from build123d import *

# Parameters (mm, degrees)
SKETCH3_W                       = 3
SKETCH3_H                       = 10
BOSS_EXTRUDE1_DEPTH             = 15
SKETCH3_W_2                     = 9.160158842
BOSS_EXTRUDE1_2_DEPTH           = 15
BOSS_EXTRUDE1_3_DEPTH           = 15
SKETCH4_W                       = 22.820603272
SKETCH4_H                       = 10
BOSS_EXTRUDE2_DEPTH             = 3
SKETCH5_W                       = 22.820603272
SKETCH5_H                       = 10
BOSS_EXTRUDE3_DEPTH             = 3
SKETCH7_W                       = 16
SKETCH7_H                       = 14.76
BOSS_EXTRUDE4_DEPTH             = 10
SKETCH8_W                       = 6.35
SKETCH8_H                       = 35.2
CUT_EXTRUDE1_DEPTH              = 10
TAP_DRILL_FOR_M3X0_5_TAP1_D     = 2.5
TAP_DRILL_FOR_M3X0_5_TAP1_DEPTH = 10
TAP_DRILL_FOR_M3X0_5_TAP1_TIP   = 0.751075774
BOSS_EXTRUDE5_DEPTH             = 10
CUT_EXTRUDE4_DEPTH              = 319.166667347
CUT_EXTRUDE5_DEPTH              = 5
M4_START                        = -10.356969024
M4_CLEARANCE_SLOT1_DEPTH        = 5
FILLET4_R                       = 2


# Read off the part's stored shape, not the designer's step: M4 Clearance Slot1
with BuildPart() as part:
    # Sketch3 → Boss-Extrude1 (new body)
    with BuildSketch(Plane(origin=(-193.9, 0, 193.9), x_dir=(0.7071067811865475, 0, 0.7071067811865477), z_dir=(-0.7071067811865477, 0, 0.7071067811865475))):
        with Locations((-9.910301636, -10.356969024)):
            Rectangle(SKETCH3_W, SKETCH3_H)
    extrude(amount=-BOSS_EXTRUDE1_DEPTH)



with BuildPart() as body_2:
    # Sketch3 → Boss-Extrude1 2 (new body)
    with BuildSketch(Plane(origin=(-193.9, 0, 193.9), x_dir=(0.7071067811865475, 0, 0.7071067811865477), z_dir=(-0.7071067811865477, 0, 0.7071067811865475))):
        with Locations((0, -10.356969024)):
            Rectangle(SKETCH3_W_2, SKETCH3_H)
    extrude(amount=-BOSS_EXTRUDE1_2_DEPTH)


with BuildPart() as body_3:
    # Sketch3 → Boss-Extrude1 3 (new body)
    with BuildSketch(Plane(origin=(-193.9, 0, 193.9), x_dir=(0.7071067811865475, 0, 0.7071067811865477), z_dir=(-0.7071067811865477, 0, 0.7071067811865475))):
        with Locations((9.910301636, -10.356969024)):
            Rectangle(SKETCH3_W, SKETCH3_H)
    extrude(amount=-BOSS_EXTRUDE1_3_DEPTH)


with BuildPart() as part_1:
    add(part.part)

    add(body_2.part)  # Boss-Extrude2 merges body 2

    add(body_3.part)  # Boss-Extrude2 merges body 3
    # Sketch4 → Boss-Extrude2 (add)
    with BuildSketch(Plane(origin=(-193.9, 0, 193.9), x_dir=(0.7071067811865472, 0, 0.7071067811865479), z_dir=(-0.7071067811865479, 0, 0.7071067811865472))):
        with Locations((0, -10.356969024)):
            Rectangle(SKETCH4_W, SKETCH4_H)
    extrude(amount=BOSS_EXTRUDE2_DEPTH)

    # Sketch5 → Boss-Extrude3 (add)
    with BuildSketch(Plane(origin=(-183.293398282, 0, 183.293398282), x_dir=(-0.7071067811865472, 0, -0.7071067811865479), z_dir=(0.7071067811865479, 0, -0.7071067811865472))):
        with Locations((0, -10.356969024)):
            Rectangle(SKETCH5_W, SKETCH5_H)
    extrude(amount=BOSS_EXTRUDE3_DEPTH)

    # Sketch7 → Boss-Extrude4 (add)
    # profile 1 of 2: a face of its own
    with BuildSketch(Plane(origin=(0, -5.356969024, 0), x_dir=(1, 0, 0), z_dir=(0, 1, 0))):
        Polygon((-204.089622006, -203.8), (-188.242640687, -203.8), (-204.089622006, -187.953018681), align=None)
    # profile 2 of 2: a face of its own
    with BuildSketch(Plane(origin=(0, -5.356969024, 0), x_dir=(1, 0, 0), z_dir=(0, 1, 0))):
        Polygon((-183.9, -239), (-186.9, -239), (-186.9, -243.88), (-147.3, -243.88), (-147.3, -173.103776276), (-189.240379601, -173.103776276), (-173.103776276, -189.240379601), (-187.663396675, -203.8), (-183.9, -203.8), align=None)
        with Locations((-158.3, -233.5)):
            Rectangle(SKETCH7_W, SKETCH7_H, mode=Mode.SUBTRACT)
    extrude(amount=-BOSS_EXTRUDE4_DEPTH)

    # Sketch8 → Cut-Extrude1 (cut)
    with BuildSketch(Plane(origin=(0, -5.356969024, 0), x_dir=(1, 0, 0), z_dir=(0, 1, 0))):
        Polygon((-188.242640687, -203.8), (-187.953018681, -204.089622006), (-187.663396675, -203.8), align=None)
        with Locations((-180.725, -221.4)):
            Rectangle(SKETCH8_W, SKETCH8_H)
    extrude(amount=-CUT_EXTRUDE1_DEPTH, mode=Mode.SUBTRACT)

    # Tap Drill for M3x0.5 Tap1
    with Locations(Plane.ZY.offset(177.55)):
        with Locations((211.9, -10.356969024), (231.9, -10.356969024), (221.9, -10.356969024)):
            Hole(TAP_DRILL_FOR_M3X0_5_TAP1_D / 2, depth=TAP_DRILL_FOR_M3X0_5_TAP1_DEPTH)
            with Locations((0, 0, -(TAP_DRILL_FOR_M3X0_5_TAP1_DEPTH + TAP_DRILL_FOR_M3X0_5_TAP1_TIP / 2))):  # 118° drill point
                Cone(0, TAP_DRILL_FOR_M3X0_5_TAP1_D / 2, TAP_DRILL_FOR_M3X0_5_TAP1_TIP, mode=Mode.SUBTRACT)

    # Sketch13 → Boss-Extrude5 (add)
    with BuildSketch(Plane(origin=(0, -5.356969024, 0), x_dir=(1, 0, 0), z_dir=(0, 1, 0))):
        Polygon((-204.089622006, -173.103776276), (-204.089622006, -187.953018681), (-189.240379601, -173.103776276), align=None)
    extrude(amount=-BOSS_EXTRUDE5_DEPTH)

    # Sketch15 → Cut-Extrude4 (cut, through all)
    with BuildSketch(Plane(origin=(0, -5.356969024, 0), x_dir=(1, 0, 0), z_dir=(0, 1, 0))):
        with BuildLine():
            Line((-186.532003499, -177.933472722), (-187.119059257, -177.346416963))
            ThreePointArc((-187.119059257, -177.346416963), (-188.179719429, -176.907077135), (-189.240379601, -177.346416963))
            Line((-189.240379601, -177.346416963), (-199.846981319, -187.953018681))
            ThreePointArc((-199.846981319, -187.953018681), (-200.286321147, -189.013678853), (-199.846981319, -190.074339025))
            Line((-199.846981319, -190.074339025), (-199.25992556, -190.661394783))
            ThreePointArc((-199.25992556, -190.661394783), (-198.199265388, -191.100734612), (-197.138605217, -190.661394783))
            Line((-197.138605217, -190.661394783), (-186.532003499, -180.054793066))
            ThreePointArc((-186.532003499, -180.054793066), (-186.092663671, -178.994132894), (-186.532003499, -177.933472722))
        make_face()
        with BuildLine():
            Line((-177.346416963, -187.119059257), (-177.933472722, -186.532003499))
            ThreePointArc((-177.933472722, -186.532003499), (-178.994132894, -186.092663671), (-180.054793066, -186.532003499))
            Line((-180.054793066, -186.532003499), (-190.661394783, -197.138605217))
            ThreePointArc((-190.661394783, -197.138605217), (-191.100734612, -198.199265388), (-190.661394783, -199.25992556))
            Line((-190.661394783, -199.25992556), (-190.074339025, -199.846981319))
            ThreePointArc((-190.074339025, -199.846981319), (-189.013678853, -200.286321147), (-187.953018681, -199.846981319))
            Line((-187.953018681, -199.846981319), (-177.346416963, -189.240379601))
            ThreePointArc((-177.346416963, -189.240379601), (-176.907077135, -188.179719429), (-177.346416963, -187.119059257))
        make_face()
    extrude(amount=-CUT_EXTRUDE4_DEPTH, mode=Mode.SUBTRACT)

    # Sketch16 → Cut-Extrude5 (cut)
    with BuildSketch(Plane.XZ.offset(15.356969024)):
        Polygon((-187.119059257, 177.346416963), (-177.346416963, 187.119059257), (-190.074339025, 199.846981319), (-199.846981319, 190.074339025), align=None)
    extrude(amount=-CUT_EXTRUDE5_DEPTH, mode=Mode.SUBTRACT)

    # M4 Clearance Slot1 outline → M4 Clearance Slot1 (cut)
    with BuildSketch(Plane(origin=(0, 0, 0), x_dir=(1, 0, 0), z_dir=(0, 1, 0)).offset(M4_START)):
        with BuildLine():
            Line((-188.419922446, -185.23794193), (-191.955456352, -188.773475836))
            ThreePointArc((-191.955456352, -188.773475836), (-191.955456352, -191.955456352), (-188.773475836, -191.955456352))
            Line((-188.773475836, -191.955456352), (-185.23794193, -188.419922446))
            ThreePointArc((-185.23794193, -188.419922446), (-185.23794193, -185.23794193), (-188.419922446, -185.23794193))
        make_face()
    extrude(amount=M4_CLEARANCE_SLOT1_DEPTH, mode=Mode.SUBTRACT)

    # Fillet4
    fillet4_edges = [part_1.edges().sort_by_distance(p)[0] for p in [
        (-166.3, -10.356969024, 240.88),
        (-166.3, -10.356969024, 226.12),
        (-150.3, -10.356969024, 226.12),
        (-150.3, -10.356969024, 240.88),
    ]]
    fillet(fillet4_edges, radius=FILLET4_R)


solid = part_1.part
Geometry check sheet. Reference: the model listing, model coordinates, mm. A direction names the side the tool comes from. Give positions to 0.01 mm unless a question says otherwise; leave off trailing zeros. Order: outer loops, then holes, each group sorted by start corner. A loop starts at its lowest first (then second) coordinate and runs counter-clockwise, first axis right, second up. Notation, with made-up numbers: (-39.5, -34.5) - (-10.5, -34.5) arc R31 ccw to (-10.5, -5.5) - close; hole circle Ø4 at (77, -24). An arc over 180 degrees is marked (long way). Answer as a JSON object with one key per item and string values.
(1) Tool access check on faces 3 (the cylindrical face through (-172.48, -10.836, 210.745)), 4 (the cylindrical face through (-191.1, -7.8, 198.2)), 5 (the flat face through (-186.9, -10, 241)). Record the directions out of +Z, -Z, +X, -X, +Y, -Y that give a thin tool (end or side, any length) a straight path to the whole face; none if there is none.
Report:
{"face 3": "-X", "face 4": "+Y, -Y", "face 5": "+Z, -X, +Y, -Y"}
(2) Draft check along Y on faces 1 (the cylindrical face through (-172.48, -10.836, 220.745)), 2 (the flat face through (-182.724, -10.427, 194.618)). Enter one of: released by +Y, released by -Y, zero draft, split by the parting line, or undercut.
Report:
{"face 1": "undercut", "face 2": "zero draft"}
(3) Depth check by flat-ended pin: pin 1 Ø5 at (y, z) = (-11, 236) entering from -X; pin 2 Ø2.5 at (y, z) = (-12.5, 242.5) entering from -X; pin 3 Ø5 at (x, y) = (-191.5, -10.5) entering from +Z; pin 4 Ø17 at (x, z) = (-184, 190) entering from -Y. Enter the tip coordinate at first touch or a pass-through.
Report:
{"pin 1": "x = -177.55", "pin 2": "x = -186.9", "pin 3": "z = 203.8", "pin 4": "y = -15.36"}
(4) Cross-section at A-A (z = 229). Record the cut outline in (x, y).
Report:
{"outline": "(-177.55, -15.36) - (-166.3, -15.36) - (-166.3, -5.36) - (-177.55, -5.36) - close; (-150.3, -15.36) - (-147.3, -15.36) - (-147.3, -5.36) - (-150.3, -5.36) - close"}
(5) Cross-section at C-C (x = -173). Record the cut outline in (y, z).
Report:
{"outline": "(-15.36, 173.1) - (-5.36, 173.1) - (-5.36, 243.88) - (-15.36, 243.88) - close; hole circle Ø2.5 at (-10.36, 211.9); hole circle Ø2.5 at (-10.36, 221.9); hole circle Ø2.5 at (-10.36, 231.9)"}
(6) Cross-section at D-D (x = -159.5). Record the cut outline in (y, z), then the cut area to 3 significant figures.
Report:
{"outline": "(-15.36, 173.1) - (-5.36, 173.1) - (-5.36, 226.12) - (-15.36, 226.12) - close; (-15.36, 240.88) - (-5.36, 240.88) - (-5.36, 243.88) - (-15.36, 243.88) - close", "area": "560 mm^2"}
(7) Material ranges on line 1 (X direction, y = -10.25, z = 189.5); line 2 (Z direction, x = -192, y = -10.25); line 3 (Z direction, x = -156, y = -7.5), recorded low to high.
Report:
{"line 1": "-204.09 to -200.21, -195.98 to -192.44, -186.32 to -183.02, -177.61 to -147.3", "line 2": "173.1 to 180.11, 185.52 to 188.82, 191.91 to 203.8", "line 3": "173.1 to 226.12, 240.88 to 243.88"}
(8) Cross-section at B-B (y = -12.75). Record the cut outline in (x, z), then the cut area to 3 significant figures.
Report:
{"outline": "(-204.09, 173.1) - (-147.3, 173.1) - (-147.3, 243.88) - (-186.9, 243.88) - (-186.9, 239) - (-177.55, 239) - (-177.55, 203.8) - (-204.09, 203.8) - close; hole (-199.85, 187.95) - (-189.24, 177.35) arc R1.5 ccw to (-187.12, 177.35) - (-177.35, 187.12) arc R1.5 ccw to (-177.35, 189.24) - (-187.95, 199.85) arc R1.5 ccw to (-190.07, 199.85) - (-199.85, 190.07) arc R1.5 ccw to start; hole (-166.3, 228.12) arc R2 ccw to (-164.3, 226.12) - (-152.3, 226.12) arc R2 ccw to (-150.3, 228.12) - (-150.3, 238.88) arc R2 ccw to (-152.3, 240.88) - (-164.3, 240.88) arc R2 ccw to (-166.3, 238.88) - close", "area": "2,470 mm^2"}
